from build123d import *

# Parameters (mm, degrees)
SKETCH1_W          = 19.05
SKETCH1_H          = 2.413
CHAMFER1_SIZE      = 0.5953125
CUT_EXTRUDE2_DEPTH = 1.79578
SKETCH6_R          = 1.833087105
CUT_EXTRUDE3_DEPTH = 1.79578
CUT_EXTRUDE3_TAPER = 45


with BuildPart() as part:
    # Sketch1 → Revolve1 (revolve)
    with BuildSketch(Plane(origin=(0, 0, 0), x_dir=(0, 0, -1), z_dir=(1, 0, 0))):
        with Locations((12.0904, 1.2065)):
            Rectangle(SKETCH1_W, SKETCH1_H)
    revolve(axis=Axis((0, 0, -21.6154), (0, 0, 1)))

    # Chamfer1
    chamfer1_edges = [part.edges().sort_by_distance(p)[0] for p in [
        (0, -2.413, -21.6154),
    ]]
    chamfer(chamfer1_edges, length=CHAMFER1_SIZE)

    # Sketch7 → Revolve2 (revolve)
    with BuildSketch(Plane(origin=(0, 0, 0), x_dir=(0, 0, -1), z_dir=(1, 0, 0)), mode=Mode.PRIVATE) as revolve2_sk:
        with BuildLine():
            Line((2.18059, 4.5847), (2.5654, 4.5847))
            Line((2.5654, 4.5847), (2.5654, 0))
            Line((2.5654, 0), (0, 0))
            Line((0, 0), (0, 2.413))
            ThreePointArc((0, 2.413), (0.925030326, 3.664791196), (2.18059, 4.5847))
        make_face()
    revolve(revolve2_sk.sketch.rotate(Axis((0, 0, 0), (0, 0, -1)), 180), axis=Axis((0, 0, 0), (0, 0, -1)))

    # Sketch5 → Cut-Extrude2 (cut)
    with BuildSketch(Plane.XY):
        Polygon((1.5875, -0.916543552), (1.5875, 0.916543552), (0, 1.833087105), (-1.5875, 0.916543552), (-1.5875, -0.916543552), (0, -1.833087105), align=None)
    extrude(amount=-CUT_EXTRUDE2_DEPTH, mode=Mode.SUBTRACT)

    # Sketch6 → Cut-Extrude3 (cut)
    with BuildSketch(Plane.XY):
        Circle(SKETCH6_R)
    extrude(amount=-CUT_EXTRUDE3_DEPTH, taper=CUT_EXTRUDE3_TAPER, mode=Mode.SUBTRACT)


solid = part.part
The model under review builds one solid part; all positions refer to its coordinate system, in mm. A direction names the side the tool comes from. Coordinates: 2 decimals unless noted, no trailing zeros. Write each loop counter-clockwise with the first axis right and the second up, starting at its lowest first coordinate (ties: lowest second). Pieces come first, ordered by that corner, then holes. Notation, with made-up numbers: (88, 89.5) - (116, 89.5) arc R18 cw to (116, 95.5) - close; hole circle Ø10 at (62, 16). An arc over 180 degrees is marked (long way). Answer as CSV lines item,"result".
(1) Mouldability with a two-part tool opening along X and no side actions: class faces 1 (the conical face through (0.865, 1.473, -0.125)), 2 (the flat face through (-2, 0, 0)), 3 (the cylindrical face through (4.476, 0.994, -2.376)) as pulls with the +X half, pulls with the -X half, needs draft (parallel to the pull), parting line crosses it, or undercut.
Data:
face 1,"undercut"
face 2,"needs draft"
face 3,"parting line crosses it"
(2) We need section B-B (z = -5.75). Give the boundary of the cut face in (x, y).
Data:
outline,"circle Ø4.83 at (0, 0)"
(3) We need section C-C (x = -3.75). Give the boundary of the cut face in (y, z), plus the area to 3 significant figures.
Data:
outline,"(-2.64, -2.57) - (2.64, -2.57) - (2.64, -2.18) arc R3.56 ccw to (-2.64, -2.18) - close"
area,"6.29 mm2"
(4) We need section A-A (y = 0). Give the boundary of the cut face in (x, z), plus the area to 3 significant figures.
Data:
outline,"(-4.58, -2.57) - (-2.41, -2.57) - (-2.41, -21.02) - (-1.82, -21.62) - (1.82, -21.62) - (2.41, -21.02) - (2.41, -2.57) - (4.58, -2.57) - (4.58, -2.18) arc R5.17 ccw to (2.41, 0) - (1.83, 0) - (1.59, -0.25) - (1.59, -1.8) - (-1.59, -1.8) - (-1.59, -0.25) - (-1.83, 0) - (-2.41, 0) arc R5.17 ccw to (-4.58, -2.18) - close"
area,"106 mm2"
(5) For line 1 along X through (y, z) = (0, -11.5); line 2 along Z through (x, y) = (-2.5, -1); line 3 along Z through (x, y) = (0.5, -2), list the stretches that pass through material, from the lowest coordinate up. Write a range as [from, to].
Data:
line 1,"x = [-2.41, 2.41]"
line 2,"z = [-2.57, -0.16]"
line 3,"z = [-21.37, 0]"
(6) We need section D-D (y = 3). Give the boundary of the cut face in (x, z), plus the area to 3 significant figures.
Data:
outline,"(-3.47, -2.57) - (3.47, -2.57) - (3.47, -2.18) arc R4.21 ccw to (-3.47, -2.18) - close"
area,"11.5 mm2"
(7) Tool access review of faces 4 (the flat face through (2, -2, -2.565)), 5 (the flat face through (-0.8, -1.37, -0.89)), 6 (the flat face through (0, 0, -21.615)): name each direction out of +Z, -Z, +X, -X, +Y, -Y from which nothing blocks a thin tool from reaching the whole face with its end or side.
Data:
face 4,"-Z"
face 5,"+Z"
face 6,"-Z, +X, -X, +Y, -Y"
(8) Clearance check with flat-ended pins moving along their axes: pin 1 Ø3 at (x, z) = (-1, -8.5) entering from +Y; pin 2 Ø1 at (x, y) = (-0.5, 0) entering from +Z; pin 3 Ø1.4 at (y, z) = (0.5, -1) entering from -X. State where each tip first meets the part, or that it passes through.
Data:
pin 1,"stops at y = 2.41"
pin 2,"stops at z = -1.8"
pin 3,"stops at x = -4.28"
